from build123d import *


with BuildPart() as part:
    # Esboço1 → Revolução1 (revolve)
    with BuildSketch(Plane(origin=(0, 0, 0), x_dir=(0, 0, -1), z_dir=(1, 0, 0)), mode=Mode.PRIVATE) as revolu_o1_sk:
        with BuildLine():
            Line((5, 30.5), (3, 30.5))
            ThreePointArc((3, 30.5), (0.878679656, 29.621320344), (0, 27.5))
            Line((0, 27.5), (0, 24.5))
            ThreePointArc((0, 24.5), (0.878679656, 22.378679656), (3, 21.5))
            Line((3, 21.5), (40, 21.5))
            Line((40, 21.5), (40, 23))
            Line((40, 23), (3, 23))
            ThreePointArc((3, 23), (1.939339828, 23.439339828), (1.5, 24.5))
            Line((1.5, 24.5), (1.5, 27.5))
            ThreePointArc((1.5, 27.5), (1.939339828, 28.560660172), (3, 29))
            Line((3, 29), (5, 29))
            Line((5, 29), (5, 30.5))
        make_face()
    revolve(revolu_o1_sk.sketch.rotate(Axis((0, 0, 0), (0, 0, 1)), 90), axis=Axis((0, 0, 0), (0, 0, 1)))


solid = part.part
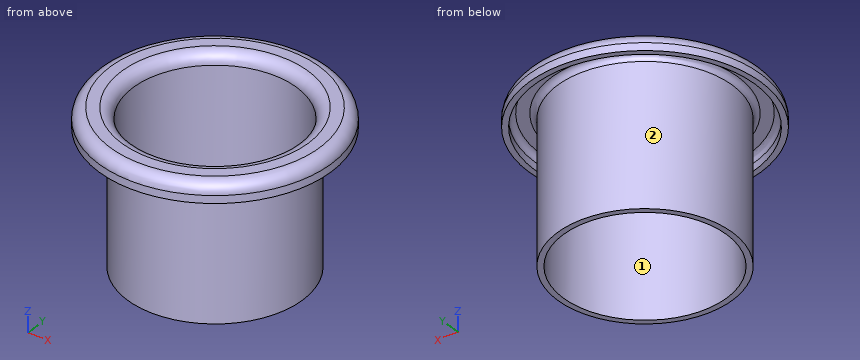
Verification items for the finished model (mm, model axes). Face numbers are marked on the shaded views. A direction names the side the tool comes from. Coordinates: 2 decimals unless noted, no trailing zeros. Order: outer loops, then holes, each group sorted by start corner. A loop starts at its lowest first (then second) coordinate and runs counter-clockwise, first axis right, second up. Notation, with made-up numbers: M 81,-26 L 137,-26 A18 ccw 137,1 Z; hole C 53.25,14.5 d1. An arc over 180 degrees is marked long. Return JSON: item names as keys, results as strings.
1) Cross-section at C-C, the plane z = -4. Record the boundary of the cut face in (x, y).
Answer list:
{"outline": "C 0,0 d61; C 0,0 d46; hole C 0,0 d58; hole C 0,0 d43"}
2) Cross-section at D-D, the plane z = -20. Record the boundary of the cut face in (x, y).
Answer list:
{"outline": "C 0,0 d46; hole C 0,0 d43"}
3) Access from +Z, -Z, +X, -X, +Y, -Y to the whole of each face (thin tool, end or side, straight path). Record for the marked faces 1 and 2.
Answer list:
{"face 1": "+Z, -Z", "face 2": "-Z"}
4) Cross-section at A-A, the plane x = 0. Record the boundary of the cut face in (y, z), and give its area (3 significant figures).
Answer list:
{"outline": "M -30.5,-5 L -29,-5 L -29,-3 A1.5 cw -27.5,-1.5 L -24.5,-1.5 A1.5 cw -23,-3 L -23,-40 L -21.5,-40 L -21.5,-3 A3 ccw -24.5,0 L -27.5,0 A3 ccw -30.5,-3 Z; M 21.5,-40 L 23,-40 L 23,-3 A1.5 cw 24.5,-1.5 L 27.5,-1.5 A1.5 cw 29,-3 L 29,-5 L 30.5,-5 L 30.5,-3 A3 ccw 27.5,0 L 24.5,0 A3 ccw 21.5,-3 Z", "area": "147 mm2"}
5) Gauge pin test, flat ends, axial feed: pin 1 (3 mm diameter, centred on y = 15, z = -33, fed in from -X); pin 2 (10 mm diameter, centred on y = 9, z = -14, fed in from +X); pin 3 (10 mm diameter, centred on y = 23, z = -22.5, fed in from -X). Record the tip position at first contact, or that the pin passes through.
Answer list:
{"pin 1": "x = -18.62", "pin 2": "x = 22.65", "pin 3": "x = -14.32"}
6) Thickness scan on L1, parallel to Y at x = 0, z = -3.9; L2, parallel to X at y = 12, z = -3; L3, parallel to Y at x = 0, z = -13. Record the ranges inside material, lowest first. Write a range as [from, to].
Answer list:
{"L1": "[-30.5, -29], [-23, -21.5], [21.5, 23], [29, 30.5]", "L2": "[-28.04, -26.4], [-19.62, -17.84], [17.84, 19.62], [26.4, 28.04]", "L3": "[-23, -21.5], [21.5, 23]"}
